Autodesk Inventor part; units mm, degrees
ref_plane "YZ Plane" through (0, 0, 0) normal (1, 0, 0) x (0, 1, 0)
ref_plane "XZ Plane" through (0, 0, 0) normal (0, 1, 0) x (-1, 0, 0)
ref_plane "XY Plane" through (0, 0, 0) normal (0, 0, 1) x (1, 0, 0)
sketch "スケッチ4" plane through (0, 0, 0) normal (0, 1, 0) x (-1, 0, 0)
  line L0 (0, 0) -> (-30, 0)
  line L1 (-30, 0) -> (-30, -30)
  line L2 (-30, -30) -> (0, -30)
  line L3 (0, -30) -> (0, 0)
  dimension "d6" = 30
  dimension "d7" = 30
extrude "押し出し2" add sketch "スケッチ4" along normal blind 26.7
sketch "スケッチ5" plane through (0, 26.7, 0) normal (0, 1, 0) x (1, 0, 0)
  circle A0 centre (15, 15) radius 12.95
  line L0 (0, 30) -> (0, 0)
  line L1 (30, 30) -> (0, 30)
  line L2 (7.75, 4.2697) -> (22.25, 4.2697)
  line L3 (22.25, 4.2697) -> (22.25, -0.093)
  line L4 (22.25, -0.093) -> (7.75, -0.093)
  line L5 (7.75, -0.093) -> (7.75, 4.2697)
  point P0 (0, 15)
  point P1 (15, 30)
  point P2 (7.75, 2.0883)
  point P3 (22.25, 4.2697)
  dimension "d10" = 25.9
  dimension "d28" = 14.5
  dimension "d29" = 7.25
sketch "スケッチ6" plane through (0, 26.7, 0) normal (0, 1, 0) x (1, 0, 0)
  circle A0 centre (15, 15) radius 12.95
  line L0 (30, 0) -> (30, 30) construction
  line L1 (30, 30) -> (0, 30) construction
  line L2 (0, 0) -> (30, 0) construction
  circle A1 centre (24.5802, 2.4198) radius 0 construction
  circle A2 centre (15, 15) radius 16 construction
  line L3 (30, 0) -> (0, 30) construction
  line L4 (0, 30) -> (0, 0) construction
  line L5 (0, 0) -> (30, 30) construction
  point P0 (24.5802, 2.4198)
  point P1 (3.6863, 3.6863)
  point P2 (3.6863, 26.3137)
  point P3 (26.3137, 26.3137)
  point P4 (26.3137, 3.6863)
  dimension "d61" = 32
fillet "フィレット1" radius 2 4 edges at (0, 13.35, -30) (0, 13.35, 0) (30, 13.35, 0) (30, 13.35, -30)
extrude "押し出し3" cut sketch "スケッチ5" against normal blind 1.6
sketch "スケッチ7" plane through (0, 0, 0) normal (0, -1, 0) x (1, 0, 0)
  line L0 (0, -28) -> (0, -2)
  line L1 (28, -30) -> (2, -30)
  point P0 (0, 0)
  point P1 (15, -15)
  point P2 (0, -15)
  point P3 (15, -30)
hole "穴3" at (15, 0, -15) direction (0, 1, 0) diameter 10.7 end through all
sketch "スケッチ8" plane through (0, 0, 0) normal (0, -1, 0) x (1, 0, 0)
  line L0 (0, -28) -> (0, -2)
  line L1 (28, -30) -> (2, -30)
  circle A0 centre (15, -15) radius 9
  point P0 (0, 0)
  point P1 (0, -15)
  point P2 (15, -30)
  point P3 (15, -24)
  point P4 (6, -15)
  point P5 (15, -6)
  point P6 (24, -15)
  dimension "d39" = 18
hole "穴4" at (15, 0, -15) at (15, 0, -24) at (6, 0, -15) at (15, 0, -6) at (24, 0, -15) direction (0, 1, 0) diameter 3.2 end through all
sketch "スケッチ9" plane through (0, 25.1, 0) normal (0, 1, 0) x (1, 0, 0)
  circle A0 centre (15, 6) radius 1.6
  circle A1 centre (6, 15) radius 1.6
  circle A2 centre (15, 24) radius 1.6
  circle A3 centre (24, 15) radius 1.6
  point P0 (0, 0)
hole "穴5" at (15, 25.1, -6) at (6, 25.1, -15) at (15, 25.1, -24) at (24, 25.1, -15) direction (0, -1, 0) diameter 6 depth 15 tip angle 118
sketch "スケッチ10" plane through (0, 26.7, 0) normal (0, 1, 0) x (1, 0, 0)
  circle A0 centre (24.5802, 2.4198) radius 1.1
  circle A1 centre (2.4198, 2.4198) radius 1.1
  circle A2 centre (2.4198, 24.5802) radius 1.1
  circle A3 centre (24.5802, 24.5802) radius 1.1
  point P0 (0, 0)
hole "穴6" [suppressed]
hole "穴7" at (3.6863, 26.7, -3.6863) at (3.6863, 26.7, -26.3137) at (26.3137, 26.7, -26.3137) at (26.3137, 26.7, -3.6863) direction (0, -1, 0) diameter 3.2 end through all
sketch "スケッチ11" plane through (0, 25.1, 0) normal (0, 1, 0) x (1, 0, 0)
  line L0 (7.75, 0) -> (7.75, 4.2697)
  line L1 (22.25, 0) -> (7.75, 0)
  line L2 (7.75, 0) -> (7.75, 2)
  line L3 (7.75, 2) -> (22.25, 2)
  line L4 (22.25, 2) -> (22.25, 0)
  dimension "d72" = 2
extrude "押し出し5" cut sketch "スケッチ11" against normal blind 1.5
properties part number "NewPart1_ver6"
Geometry: final body of the model. Coordinates: model frame, mm. A direction names the side the tool comes from. Give positions to 0.01 mm unless a question says otherwise; leave off trailing zeros. Loops run counter-clockwise (first coordinate to the right, second up) from the corner with the lowest first, then second, coordinate; pieces in that order, holes last. Notation, with made-up numbers: (51.25, -19) - (59.25, -19) arc R29 cw to (59.25, 18) - close; hole circle Ø11 at (19.5, 12.5). An arc over 180 degrees is marked (long way). Answer as CSV lines item,"result". Start each with the question number.
(1) Section query A-A (z = -15). Output: boundary loops of the cut face in (x, y), and give its area (3 significant figures).
(2) Pin query (flat end, axial travel): P1, Ø7, axis at x = 15, z = -6, coming from the +Y side; P2, Ø1.6, axis at x = 13, z = -0.5, coming from the +Y side; P3, Ø5.5, axis at x = 24, z = -15, coming from the +Y side. Return the tip coordinate at first contact, or that it passes through.
(3) Reachability of faces 4 (the face through (15, 23.6, -1)), 5 (the face through (15, 13, 0)), 6 (the face through (17.93, 17.5, -24.65)) from +Z, -Z, +X, -X, +Y, -Y: full face, straight path, thin tool, end or side. Return the list, or none.
(4) Section query B-B (x = 15). Output: boundary loops of the cut face in (y, z).
(5) Section query C-C (z = -19.5). Output: boundary loops of the cut face in (x, y), and give its area (3 significant figures).
(6) Mould query, pull axis Z, two halves, no side actions, for faces 1 (the face through (0.6, 13.54, -29.43)), 2 (the face through (15.2, 26.7, -28.1)), 3 (the face through (15.46, 25.91, -27.94)). Classes: +Z half, -Z half, draft (parallel to the pull), parting line (faces both ways), or undercut.
(7) Ray query, line 1 along Z through (x, y) = (15, 8.75); line 2 along Z through (x, y) = (15, 14.75); line 3 along X through (y, z) = (5, -6). Return the intervals inside material, ascending. Write a range as [from, to].
(8) Section query D-D (y = 3.75). Give the number of separate pieces and of enclosed holes in the cut face, and give its area (3 significant figures).
Worked answers:
1,outline,"(0, 0) - (4.4, 0) - (4.4, 9.26) - (3, 10.1) - (3, 25.1) - (2.05, 25.1) - (2.05, 26.7) - (0, 26.7) - close; (7.6, 0) - (9.65, 0) - (9.65, 25.1) - (9, 25.1) - (9, 10.1) - (7.6, 9.26) - close; (20.35, 0) - (22.4, 0) - (22.4, 9.26) - (21, 10.1) - (21, 25.1) - (20.35, 25.1) - close; (25.6, 0) - (30, 0) - (30, 26.7) - (27.95, 26.7) - (27.95, 25.1) - (27, 25.1) - (27, 10.1) - (25.6, 9.26) - close"
1,area,"244 mm^2"
2,P1,"stops at y = 25.1"
2,P2,"stops at y = 23.6"
2,P3,"stops at y = 9.95"
3,face 4,"+Z, +Y"
3,face 5,"+Z, +X, -X, +Y, -Y"
3,face 6,"+Y"
4,outline,"(0, -30) - (26.7, -30) - (26.7, -27.95) - (25.1, -27.95) - (25.1, -27) - (10.1, -27) - (9.26, -25.6) - (0, -25.6) - close; (0, -22.4) - (9.26, -22.4) - (10.1, -21) - (25.1, -21) - (25.1, -20.35) - (0, -20.35) - close; (0, -9.65) - (25.1, -9.65) - (25.1, -9) - (10.1, -9) - (9.26, -7.6) - (0, -7.6) - close; (0, -4.4) - (9.26, -4.4) - (10.1, -3) - (25.1, -3) - (25.1, -2) - (23.6, -2) - (23.6, 0) - (0, 0) - close"
5,outline,"(0, 0) - (12.11, 0) - (12.11, 25.1) - (2.86, 25.1) - (2.86, 26.7) - (0, 26.7) - close; (17.89, 0) - (30, 0) - (30, 26.7) - (27.14, 26.7) - (27.14, 25.1) - (17.89, 25.1) - close"
5,area,"617 mm^2"
6,face 1,"-Z half"
6,face 2,"draft"
6,face 3,"undercut"
7,line 1,"z = [-30, -25.6], [-22.4, -20.35], [-9.65, -7.6], [-4.4, 0]"
7,line 2,"z = [-30, -27], [-21, -20.35], [-9.65, -9], [-3, 0]"
7,line 3,"x = [0, 13.4], [16.6, 30]"
8,separate pieces,"1"
8,enclosed holes,"9"
8,area,"742 mm^2"
